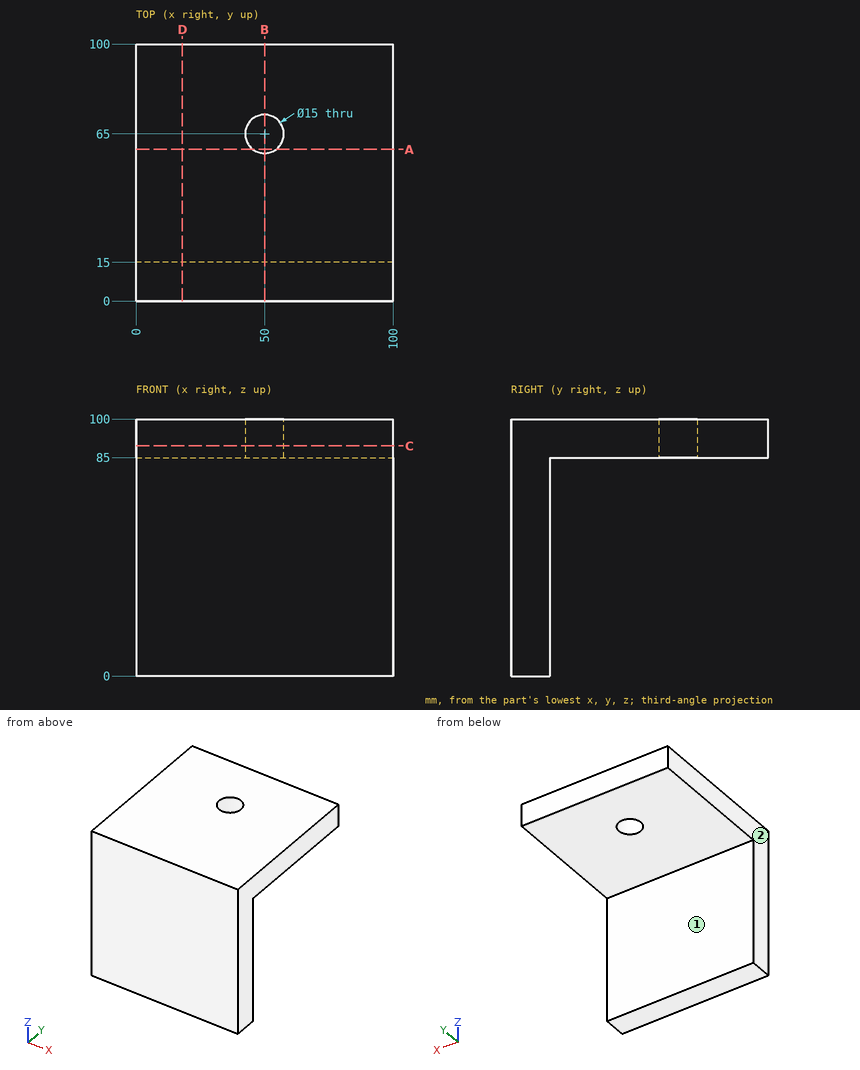
Print and shaded views of the part. All mm, measured from the part's lowest x, y and z. A direction names the side the tool comes from. Round coordinates to 2 decimals unless told otherwise and drop trailing zeros. Order: outer loops, then holes, each group sorted by start corner. A loop starts at its lowest first (then second) coordinate and runs counter-clockwise, first axis right, second up.
Q1. Which spindle directions (+Z, -Z, +X, -X, +Y, -Y) get a long thin tool onto all of the face, cutting with end or side? Do the marked faces 1 and 2. Say none if no direction does.
Q2. Wall check: L1, parallel to Y at x = 50, z = 89.5; L2, parallel to Z at x = 13, y = 79.5; L3, parallel to Y at x = 42.5, z = 81. Give the ranges that are in metal, low to high.
Q3. Slice it at D-D (x = 18). Write the cut outline in (y, z), and give its area (4 significant figures).
Q4. Drop flat-ended pins along their axis: pin 1 (1.5 mm diameter, centred on x = 73, z = 32.5, fed in from +Y); pin 2 (4 mm diameter, centred on x = 90, y = 50, fed in from -Z). Give the stop position or say it passes through.
Q5. Slice it at C-C (z = 89.5). Write the cut outline in (x, y), and give its area (3 significant figures).
Q6. Slice it at B-B (x = 50). Write the cut outline in (y, z), and give its area (3 significant figures).
Q7. Slice it at A-A (y = 59). Write the cut outline in (x, z).
Results below:
1. face 1: -Z, +X, -X, +Y
1. face 2: +Z, -Z, -X, +Y, -Y
2. L1: y = 0 to 57.5, 72.5 to 100
2. L2: z = 85 to 100
2. L3: y = 0 to 15
3. outline: (0, 0) - (15, 0) - (15, 85) - (100, 85) - (100, 100) - (0, 100) - close
3. area: 2,775 mm2
4. pin 1: stops at y = 15
4. pin 2: stops at z = 85
5. outline: (0, 0) - (100, 0) - (100, 100) - (0, 100) - close; hole circle Ø15 at (50, 65)
5. area: 9,820 mm2
6. outline: (0, 0) - (15, 0) - (15, 85) - (57.5, 85) - (57.5, 100) - (0, 100) - close; (72.5, 85) - (100, 85) - (100, 100) - (72.5, 100) - close
6. area: 2,550 mm2
7. outline: (0, 85) - (45.5, 85) - (45.5, 100) - (0, 100) - close; (54.5, 85) - (100, 85) - (100, 100) - (54.5, 100) - close
